The listing builds one solid part. Answer for the finished solid, in the listing's coordinates (mm). Face numbers are marked on the shaded views. A direction names the side the tool comes from. Round coordinates to 2 decimals unless told otherwise and drop trailing zeros. Order: outer loops, then holes, each group sorted by start corner. A loop starts at its lowest first (then second) coordinate and runs counter-clockwise, first axis right, second up. Notation, with made-up numbers: (43.25, 15.25) -> (88.25, 15.25) arc R22 cw to (88.25, 38.25) -> close; hole circle Ø2 at (35.25, -17). An arc over 180 degrees is marked (long way). Return JSON: item names as keys, results as strings. Group by question number.
(1) The part is cut by section C-C (z = -2.5). Determine the outline of the cut face in (x, y), plus the area to 3 significant figures.
(2) Determine the mould class of the marked faces 1, 2 and 3 for opening direction X: +X half, -X half, draft (parallel to the pull), parting line (faces both ways), or undercut.
(3) Each of these flat-tipped pins is pushed along its axis until it touches: pin 1 (1 mm diameter, centred on y = -7, z = 2, fed in from +X); pin 2 (1 mm diameter, centred on x = -8, z = -2.5, fed in from -Y); pin 3 (6 mm diameter, centred on x = -6.5, y = -3.5, fed in from +Z); pin 4 (8 mm diameter, centred on x = 1.5, y = -7, fed in from +Z). Where does it stop, or does it pass through?
(4) Consider line 1 (X direction, y = 0, z = 0.5); line 2 (Z direction, x = -4.75, y = -6.25). Determine where each line is inside the solid, lowest interval first. Write a range as [from, to].
(5) Which of the six approach directions +Z, -Z, +X, -X, +Y, -Y give full straight-line access (tool end or side, diameter ignored) to the marked faces 4, 5 and 6?
(6) The part is cut by section A-A (y = 0). Determine the outline of the cut face in (x, z).
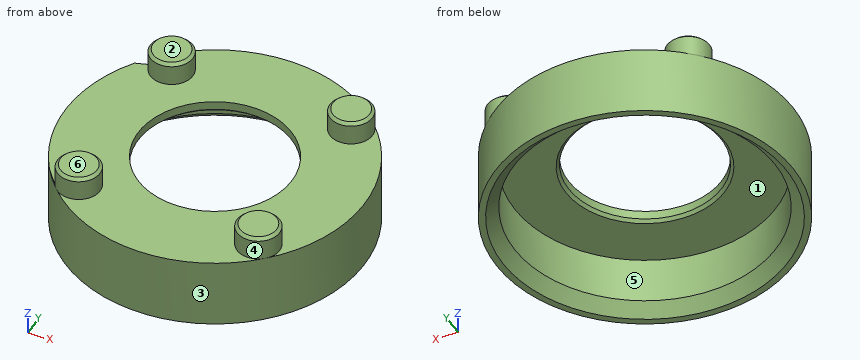
from build123d import *

# Parameters (mm, degrees)
SKETCH1_R           = 12.6
SKETCH1_R_2         = 11.1
BOSS_EXTRUDE1_DEPTH = 5
CHAMFER1_SIZE       = 1
SKETCH2_R           = 1.8
BOSS_EXTRUDE2_DEPTH = 3
BOSS_EXTRUDE3_START = 1
SKETCH3_R           = 12.6
BOSS_EXTRUDE3_DEPTH = 1
SKETCH5_R           = 6.5
CUT_EXTRUDE1_DEPTH  = 19.507295859
CHAMFER2_SIZE       = 0.25
CHAMFER3_SIZE       = 0.25
BOSS_EXTRUDE4_START = -6
SKETCH7_R           = 12.65
SKETCH7_R_2         = 12.6
BOSS_EXTRUDE4_DEPTH = 6


with BuildPart() as part:
    # Sketch1 → Boss-Extrude1 (new body)
    with BuildSketch(Plane.XY):
        Circle(SKETCH1_R)
        Circle(SKETCH1_R_2, mode=Mode.SUBTRACT)
    extrude(amount=-BOSS_EXTRUDE1_DEPTH)

    # Chamfer1
    chamfer1_edges = [part.edges().sort_by_distance(p)[0] for p in [
        (-11.1, 0, -5),
    ]]
    chamfer(chamfer1_edges, length=CHAMFER1_SIZE)

    # Sketch2 → Boss-Extrude2 (add)
    with BuildSketch(Plane.XY):
        with Locations(Location((7.672108576, -7.672108576, 0), (0, 0, 228.298602852))):
            Circle(SKETCH2_R)
        with Locations(Location((-7.672108576, -7.672108576, 0), (0, 0, 210.392900991))):
            Circle(SKETCH2_R)
        with Locations(Location((-7.672108576, 7.672108576, 0), (0, 0, 149.607099009))):
            Circle(SKETCH2_R)
        with Locations(Location((7.672108576, 7.672108576, 0), (0, 0, 131.701397148))):
            Circle(SKETCH2_R)
    extrude(amount=BOSS_EXTRUDE2_DEPTH)

    # Sketch3 → Boss-Extrude3 (add)
    with BuildSketch(Plane.XY.offset(BOSS_EXTRUDE3_START)):
        Circle(SKETCH3_R)
    extrude(amount=-BOSS_EXTRUDE3_DEPTH)

    # Sketch5 → Cut-Extrude1 (cut, through all)
    with BuildSketch(Plane.XY):
        Circle(SKETCH5_R)
    extrude(amount=CUT_EXTRUDE1_DEPTH, mode=Mode.SUBTRACT)

    # Chamfer2
    chamfer2_edges = [part.edges().sort_by_distance(p)[0] for p in [
        (8.869555986, -6.328189047, 3),
        (-6.119471127, -6.761440167, 3),
        (-6.119471127, 6.761440167, 3),
        (8.869555986, 6.328189047, 3),
    ]]
    chamfer(chamfer2_edges, length=CHAMFER2_SIZE)

    # Chamfer3
    chamfer3_edges = [part.edges().sort_by_distance(p)[0] for p in [
        (-6.5, 0, 0),
    ]]
    chamfer(chamfer3_edges, length=CHAMFER3_SIZE)

    # Sketch7 → Boss-Extrude4 (add)
    with BuildSketch(Plane(origin=(0, 0, -5), x_dir=(-1, 0, 0), z_dir=(0, 0, -1)).offset(BOSS_EXTRUDE4_START)):
        Circle(SKETCH7_R)
        Circle(SKETCH7_R_2, mode=Mode.SUBTRACT)
    extrude(amount=BOSS_EXTRUDE4_DEPTH)


solid = part.part
Answer below:
{
 "1": {"outline": "circle Ø25.3 at (0, 0); hole circle Ø22.2 at (0, 0)", "area": "116 mm²"},
 "2": {"face 1": "undercut", "face 2": "draft", "face 3": "parting line"},
 "3": {"pin 1": "stops at x = 9.46", "pin 2": "stops at y = -10.19", "pin 3": "stops at z = 3", "pin 4": "stops at z = 1"},
 "4": {"line 1": "x = [-12.65, -6.5], [6.5, 12.65]", "line 2": "z = [0, 1]"},
 "5": {"face 4": "+Z", "face 5": "-Z", "face 6": "+Z, +X, -X, +Y, -Y"},
 "6": {"outline": "(-12.65, -5) -> (-12.1, -5) -> (-11.1, -4) -> (-11.1, 0) -> (-6.75, 0) -> (-6.5, 0.25) -> (-6.5, 1) -> (-12.65, 1) -> close; (6.5, 0.25) -> (6.75, 0) -> (11.1, 0) -> (11.1, -4) -> (12.1, -5) -> (12.65, -5) -> (12.65, 1) -> (6.5, 1) -> close"}
}
